Autodesk Inventor part; units mm, degrees
ref_plane "YZ Plane" through (0, 0, 0) normal (1, 0, 0) x (0, 1, 0)
ref_plane "XZ Plane" through (0, 0, 0) normal (0, 1, 0) x (-1, 0, 0)
ref_plane "XY Plane" through (0, 0, 0) normal (0, 0, 1) x (1, 0, 0)
sketch "Boceto1" plane through (0, 0, 0) normal (1, 0, 0) x (0, 1, 0)
  line L0 (12, 30) -> (-12, 30)
  line L1 (-12, 30) -> (-12, -30)
  line L2 (-12, -30) -> (12, -30)
  line L3 (12, -30) -> (12, 30)
  circle A0 centre (0, 11.5) radius 9
  point P0 (0, 0)
  point P1 (12, 0)
  point P2 (0, -30)
  dimension "d0" = 60
  dimension "d1" = 24
  dimension "d2" = 18
  dimension "d3" = 18.5
extrude "Extrusión1" add sketch "Boceto1" along normal blind 20 contours A0
extrude "Extrusión2" add sketch "Boceto1" along normal blind 12.5
properties part number "Cámara"
Build history of the part. All positions in model axes, mm. A direction names the side the tool comes from. Give positions to 0.01 mm unless a question says otherwise; leave off trailing zeros. Loops run counter-clockwise (first coordinate to the right, second up) from the corner with the lowest first, then second, coordinate; pieces in that order, holes last.
1) 3-axis set-ups, long thin cutter, end or side, ignore diameter. For faces 1 (the face through (20, 0, 12)), 2 (the face through (16.197, 4.153, 19.485)): which of +Z, -Z, +X, -X, +Y, -Y reach the whole face in a straight line?
Values follow:
face 1: +Z, -Z, +X, +Y, -Y
face 2: +X
2) Probe line 1 along X through (y, z) = (-1.25, -20); line 2 along Z through (x, y) = (17, -2); line 3 along Z through (x, y) = (16, 3.5). List the from-to ranges inside material, lowest first.
Values follow:
line 1: x = 0 to 12.5
line 2: z = 2.73 to 20.27
line 3: z = 3.21 to 19.79
3) Band-saw the part on C-C on x = 13.5. List the corners of the cut face in (y, z), then the cut area to 3 significant figures.
Values follow:
outline: circle Ø18 at (0, 11.5)
area: 254 mm2
4) Band-saw the part on B-B on y = 0. List the corners of the cut face in (x, z).
Values follow:
outline: (0, -30) - (12.5, -30) - (12.5, 2.5) - (20, 2.5) - (20, 20.5) - (12.5, 20.5) - (12.5, 30) - (0, 30) - close
5) Band-saw the part on A-A on z = 11.5. List the corners of the cut face in (x, y).
Values follow:
outline: (0, -12) - (12.5, -12) - (12.5, -9) - (20, -9) - (20, 9) - (12.5, 9) - (12.5, 12) - (0, 12) - close
6) Band-saw the part on D-D on y = 9.75. List the corners of the cut face in (x, z).
Values follow:
outline: (0, -30) - (12.5, -30) - (12.5, 30) - (0, 30) - close
7) Drop flat-ended pins along their axis: P1, Ø1.5, axis at y = 2.5, z = -22.5, coming from the +X side; P2, Ø5, axis at x = 15.5, y = 6, coming from the +Z side; P3, Ø8, axis at x = 17.5, z = 1.5, coming from the -Y side. Give the stop position or say it passes through.
Values follow:
P1: stops at x = 12.5
P2: stops at z = 19.79
P3: stops at y = -6.71
